Work out the finished part from the listing and answer in its coordinate system (mm). Coordinates: 2 decimals unless noted, no trailing zeros. Order: outer loops, then holes, each group sorted by start corner. A loop starts at its lowest first (then second) coordinate and runs counter-clockwise, first axis right, second up. Notation, with made-up numbers: M -1.5,53 L 16.5,53 A19 ccw 16.5,59 Z; hole C 51,-27.75 d5. An arc over 180 degrees is marked long. Answer in a Markdown table with one row per item. Add a question column.
Item 1: Flat-ended cylindrical pins translate along their axes: pin 1 Ø4 at (x, z) = (0, 0) entering from -Y; pin 2 Ø5.5 at (x, z) = (0, 0) entering from -Y; pin 3 Ø5 at (x, y) = (5, 301.5) entering from -Z. Find the tip coordinate at first contact, or state that the pin passes through.
Item 2: Consider line 1 (Z direction, x = 0, y = -408); line 2 (X direction, y = -211, z = -0.5); line 3 (Z direction, x = -1.25, y = -180). Determine where each line is inside the solid, lowest interval first. Write a range as from..to.
Item 3: The part is cut by section A-A (y = 10). Write down the section's boundary in (x, z), then the cut area to 3 significant figures.
Autodesk Inventor part; units mm, degrees
ref_plane "YZ Plane" through (0, 0, 0) normal (1, 0, 0) x (0, 1, 0)
ref_plane "XZ Plane" through (0, 0, 0) normal (0, 1, 0) x (-1, 0, 0)
ref_plane "XY Plane" through (0, 0, 0) normal (0, 0, 1) x (1, 0, 0)
sketch "Sketch1" plane through (0, 0, 0) normal (0, 1, 0) x (-1, 0, 0)
  circle A0 centre (0, 0) radius 6.35
  dimension "d0" = 12.7
extrude "Extrusion1" add sketch "Sketch1" along normal mid plane 850.9
sketch "Sketch2" plane through (0, 425.45, 0) normal (0, 1, 0) x (1, 0, 0)
  circle A0 centre (0, 0) radius 6.35 construction
hole "Hole1" at (0, 425.45, 0) direction (0, -1, 0) diameter 4.9784 depth 19.05 tip angle 118
sketch "Sketch3" plane through (0, -425.45, 0) normal (0, -1, 0) x (1, 0, 0)
  circle A0 centre (0, 0) radius 6.35 construction
hole "Hole2" at (0, -425.45, 0) direction (0, 1, 0) diameter 4.9784 depth 38.1 tip angle 118
properties part number "EL2-025" material "Aluminum 6061"
Reply:
| question | item | result |
|---|---|---|
| 1 | pin 1 | stops at y = -387.06 |
| 1 | pin 2 | stops at y = -425.45 |
| 1 | pin 3 | stops at z = -5.84 |
| 2 | line 1 | z = -6.35..-2.49, 2.49..6.35 |
| 2 | line 2 | x = -6.33..6.33 |
| 2 | line 3 | z = -6.23..6.23 |
| 3 | outline | C 0,0 d12.7 |
| 3 | area | 127 mm2 |
